from build123d import *

# Parameters (mm, degrees)
SKETCH5_R          = 5
SKETCH5_R_2        = 2.5
CUT_EXTRUDE1_DEPTH = 50
SKETCH5_3_R        = 2.5
CUT_EXTRUDE2_DEPTH = 50


with BuildPart() as part:
    # Sketch3 → Revolve4 (revolve)
    with BuildSketch(Plane(origin=(0, 0, 0), x_dir=(0, 0, -1), z_dir=(1, 0, 0)), mode=Mode.PRIVATE) as revolve4_sk:
        with BuildLine():
            Line((40, 2), (40, 0))
            Line((40, 0), (75, 0))
            ThreePointArc((75, 0), (78.535533906, 1.464466094), (80, 5))
            Line((80, 5), (80, 165))
            ThreePointArc((80, 165), (77.47091582, 178.997516479), (70.203476621, 191.224988084))
            Line((70.203476621, 191.224988084), (67.5, 191.224988084))
            ThreePointArc((67.5, 191.224988084), (75.277471565, 179.124446892), (78, 165))
            Line((78, 165), (78, 7))
            ThreePointArc((78, 7), (76.535533906, 3.464466094), (73, 2))
            Line((73, 2), (42, 2))
            Line((42, 2), (40, 2))
        make_face()
    revolve(revolve4_sk.sketch.rotate(Axis((0, 250.694261232, -40), (0, -1, 0)), 180), axis=Axis((0, 250.694261232, -40), (0, -1, 0)))

    # Sketch5 → Cut-Extrude1 (cut)
    # profile 1 of 2: a face of its own
    with BuildSketch(Plane(origin=(0, 0, 0), x_dir=(0, 0, -1), z_dir=(1, 0, 0))):
        with Locations(Location((40, 10, 0), (0, 0, 216.869897646))):
            Circle(SKETCH5_R)
        with Locations((40, 10)):
            Circle(SKETCH5_R_2, mode=Mode.SUBTRACT)
    # profile 2 of 2: a face of its own
    with BuildSketch(Plane(origin=(0, 0, 0), x_dir=(0, 0, -1), z_dir=(1, 0, 0))):
        with Locations((40, 10)):
            Circle(SKETCH5_R_2)
    extrude(amount=CUT_EXTRUDE1_DEPTH, mode=Mode.SUBTRACT)

    # Sketch5_3 → Cut-Extrude2 (cut)
    with BuildSketch(Plane(origin=(0, 0, 0), x_dir=(0, 0, -1), z_dir=(1, 0, 0))):
        with Locations((40, 10)):
            Circle(SKETCH5_3_R)
    extrude(amount=-CUT_EXTRUDE2_DEPTH, mode=Mode.SUBTRACT)


solid = part.part
Work out the finished part from the listing and answer in its coordinate system (mm). A direction names the side the tool comes from. Round coordinates to 2 decimals unless told otherwise and drop trailing zeros. Write each loop counter-clockwise with the first axis right and the second up, starting at its lowest first coordinate (ties: lowest second). Pieces come first, ordered by that corner, then holes. Notation, with made-up numbers: (70.25, 66.5) - (107.25, 66.5) arc R19 cw to (107.25, 75.5) - close; hole circle Ø9 at (54.5, 87.5). An arc over 180 degrees is marked (long way). Answer in a Markdown table with one row per item. Add a question column.
1. The mould has two halves that part along X. Classify faces 4 (the cylindrical face through (-12.015, 86.12, -1.847)), 5 (the cylindrical face through (-38.94, 9.04, -42.31)), 6 (the cylindrical face through (23.122, 84.894, -70.156)): +X half, -X half, draft (parallel to the pull), parting line (faces both ways), or undercut.
2. Given pin 1 (8 mm diameter, centred on y = 10, z = -40, fed in from +X); pin 2 (1.5 mm diameter, centred on y = 147, z = -70, fed in from -X); pin 3 (6 mm diameter, centred on y = 169, z = -52.5, fed in from +X), each flat-ended and moving along its own axis, determine where each tip first touches the part or whether it passes through.
3. A cutting plane is placed at B-B, the plane y = 29. Determine the outline of the cut face in (x, z), and give its area (3 significant figures).
4. A cutting plane is placed at A-A, the plane x = 0. Determine the outline of the cut face in (y, z).
5. Find the intervals of material crossed by line 1 along X through (y, z) = (111, -40); line 2 along Z through (x, y) = (11, 66.5); line 3 along Y through (x, z) = (-7.5, -61), in increasing order. Write a range as from..to.
6. For faces 1 (the flat face through (0, 0, -40)), 2 (the cylindrical face through (39, 6, -37)), 3 (the flat face through (0, 2, -40)), determine the directions among +Z, -Z, +X, -X, +Y, -Y from which every point of the face is accessible in a straight line to the end or side of a thin tool.
Worked out:
| question | item | result |
|---|---|---|
| 1 | face 4 | parting line |
| 1 | face 5 | draft |
| 1 | face 6 | undercut |
| 2 | pin 1 | x = -37.79 |
| 2 | pin 2 | x = -27.28 |
| 2 | pin 3 | x = 38.7 |
| 3 | outline | circle Ø80 at (0, -40); hole circle Ø76 at (0, -40) |
| 3 | area | 490 mm^2 |
| 4 | outline | (0, -75) arc R5 ccw to (5, -80) - (165, -80) arc R40 ccw to (191.22, -70.2) - (191.22, -67.5) arc R38 cw to (165, -78) - (7, -78) arc R5 cw to (2, -73) - (2, -7) arc R5 cw to (7, -2) - (165, -2) arc R38 cw to (191.22, -12.5) - (191.22, -9.8) arc R40 ccw to (165, 0) - (5, 0) arc R5 ccw to (0, -5) - close |
| 5 | line 1 | -40..-38, 38..40 |
| 5 | line 2 | -78.46..-76.37, -3.63..-1.54 |
| 5 | line 3 | 0..2 |
| 6 | face 1 | +Z, -Z, +X, -X, -Y |
| 6 | face 2 | +X |
| 6 | face 3 | none |
